Read the model definition and answer for the solid it produces. Units are mm, in the model's axes. Face numbers are marked on the shaded views. A direction names the side the tool comes from. Give positions to 0.01 mm unless a question says otherwise; leave off trailing zeros. Loops run counter-clockwise (first coordinate to the right, second up) from the corner with the lowest first, then second, coordinate; pieces in that order, holes last. Notation, with made-up numbers: (57, 65.5) -> (112, 65.5) arc R34 cw to (112, 95.5) -> close; hole circle Ø3 at (85, -7). An arc over 180 degrees is marked (long way). Write each question's results on one line, items separated by ' | '. Start each with the question number.
Item 1: Section B-B on y = 17 is taken. Write down the section's boundary in (x, z).
Item 2: Section A-A on x = -9.25 is taken. Write down the section's boundary in (y, z), and give its area (3 significant figures).
Item 3: Section C-C on x = -4 is taken. Write down the section's boundary in (y, z).
Item 4: Section D-D on y = 26 is taken. Write down the section's boundary in (x, z).
Item 5: Each of these flat-tipped pins is pushed along its axis until it touches: P1, Ø2.5, axis at x = -15.25, y = 3.25, coming from the -Z side; P2, Ø12, axis at x = 7.25, y = -18.25, coming from the +Z side; P3, Ø17.5, axis at x = -11.5, y = 23.5, coming from the +Z side. Where does it stop, or does it pass through?
Item 6: Determine the mould class of the marked faces 3, 4, 5 and 6 for opening direction Y: +Y half, -Y half, draft (parallel to the pull), parting line (faces both ways), or undercut.
Item 7: Find the intervals of material crossed by line 1 (Y direction, x = -15, z = 5.2); line 2 (X direction, y = 20, z = 5.1); line 3 (Y direction, x = 9.25, z = 1.8), in increasing order.
Item 8: Which of the six approach directions +Z, -Z, +X, -X, +Y, -Y give full straight-line access (tool end or side, diameter ignored) to the marked faces 1 and 2?
```python
from build123d import *

# Parameters (mm, degrees)
F0_W      = 38.5
F0_H      = 68.5
F1_DEPTH  = 6
F2_W      = 16
F2_H      = 16
F3_DEPTH  = 2
F5_DEPTH  = 2
F6_R      = 7.5
F7_DEPTH  = 2
F8_R      = 2
F9_DEPTH  = 8
F10_R     = 2.5
F11_DEPTH = 25
F12_R     = 2.5
F13_DEPTH = 25


with BuildPart() as f1:
    # F0 (on Top) → F1 (new body)
    with BuildSketch(Plane.XY):
        Rectangle(F0_W, F0_H)
    extrude(amount=F1_DEPTH)

    # F2 (on face) → F3 (cut)
    with BuildSketch(Plane.XY.offset(6)):
        with Locations((-9.25, 24.2511786477)):
            Rectangle(F2_W, F2_H)
        with Locations((9.25, 24.25)):
            Rectangle(F2_W, F2_H)
    extrude(amount=-F3_DEPTH, mode=Mode.SUBTRACT)

    # F4 (on face) → F5 (cut)
    with BuildSketch(Plane.XY.offset(6)):
        with BuildLine():
            Line((15.7500000197, 13.2511786477), (-15.75, 13.2511786477))
            ThreePointArc((-15.75, 13.2511786477), (-14.6893398282, 12.8118388195), (-14.25, 11.7511786477))
            ThreePointArc((-14.25, 11.7511786477), (-14.6893398282, 10.6905184759), (-15.75, 10.2511786477))
            Line((-15.75, 10.2511786477), (15.7500000167, 10.2511786477))
            ThreePointArc((15.7500000167, 10.2511786477), (14.25, 11.7511786492), (15.7500000197, 13.2511786477))
        make_face()
        with BuildLine():
            ThreePointArc((-14.25, 11.7511786477), (-14.6893398282, 12.8118388195), (-15.75, 13.2511786477))
            ThreePointArc((-15.75, 13.2511786477), (-16.8106601718, 12.8118388195), (-17.25, 11.7511786477))
            ThreePointArc((-17.25, 11.7511786477), (-16.8106601718, 10.6905184759), (-15.75, 10.2511786477))
            ThreePointArc((-15.75, 10.2511786477), (-14.6893398282, 10.6905184759), (-14.25, 11.7511786477))
        make_face()
        with BuildLine():
            ThreePointArc((17.25, 11.7511786477), (16.8106601788, 12.8118388125), (15.7500000197, 13.2511786477))
            ThreePointArc((15.7500000197, 13.2511786477), (14.25, 11.7511786492), (15.7500000167, 10.2511786477))
            ThreePointArc((15.7500000167, 10.2511786477), (16.8106601777, 10.6905184818), (17.25, 11.7511786477))
        make_face()
    extrude(amount=-F5_DEPTH, mode=Mode.SUBTRACT)

    # F6 (on face) → F7 (cut)
    with BuildSketch(Plane.XY.offset(6)):
        with Locations((7.25, -18.25)):
            Circle(F6_R)
    extrude(amount=-F7_DEPTH, mode=Mode.SUBTRACT)

    # F8 (on face) → F9 (cut)
    with BuildSketch(Plane.XY.offset(6)):
        with Locations((-15.25, 3.2511786477)):
            Circle(F8_R)
    extrude(amount=-F9_DEPTH, mode=Mode.SUBTRACT)

    # F10 (on face) → F11 (cut)
    with BuildSketch(Plane.XY.offset(4)):
        with Locations((-9.25, 24.2511786477)):
            Circle(F10_R)
    extrude(amount=-F11_DEPTH, mode=Mode.SUBTRACT)

    # F12 (on face) → F13 (cut)
    with BuildSketch(Plane.XY.offset(4)):
        with Locations((9.25, 24.25)):
            Circle(F12_R)
    extrude(amount=-F13_DEPTH, mode=Mode.SUBTRACT)


solid = f1.part
```
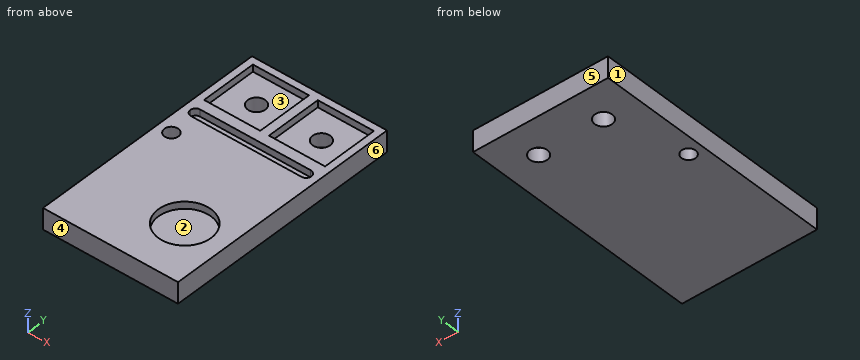
Findings:
1) outline: (-19.25, 0) -> (19.25, 0) -> (19.25, 6) -> (17.25, 6) -> (17.25, 4) -> (1.25, 4) -> (1.25, 6) -> (-1.25, 6) -> (-1.25, 4) -> (-17.25, 4) -> (-17.25, 6) -> (-19.25, 6) -> close
2) outline: (-34.25, 0) -> (21.75, 0) -> (21.75, 4) -> (16.25, 4) -> (16.25, 6) -> (13.25, 6) -> (13.25, 4) -> (10.25, 4) -> (10.25, 6) -> (-34.25, 6) -> close; (26.75, 0) -> (34.25, 0) -> (34.25, 6) -> (32.25, 6) -> (32.25, 4) -> (26.75, 4) -> close | area: 353 mm2
3) outline: (-34.25, 0) -> (34.25, 0) -> (34.25, 6) -> (32.25, 6) -> (32.25, 4) -> (16.25, 4) -> (16.25, 6) -> (13.25, 6) -> (13.25, 4) -> (10.25, 4) -> (10.25, 6) -> (-34.25, 6) -> close
4) outline: (-19.25, 0) -> (-11.04, 0) -> (-11.04, 4) -> (-17.25, 4) -> (-17.25, 6) -> (-19.25, 6) -> close; (-7.46, 0) -> (7.46, 0) -> (7.46, 4) -> (1.25, 4) -> (1.25, 6) -> (-1.25, 6) -> (-1.25, 4) -> (-7.46, 4) -> close; (11.04, 0) -> (19.25, 0) -> (19.25, 6) -> (17.25, 6) -> (17.25, 4) -> (11.04, 4) -> close
5) P1: through | P2: z = 4 | P3: z = 6
6) face 3: undercut | face 4: -Y half | face 5: +Y half | face 6: draft
7) line 1: -34.25 to 1.27, 5.24 to 10.25, 13.25 to 16.25, 32.25 to 34.25 | line 2: -19.25 to -17.25, -1.25 to 1.25, 17.25 to 19.25 | line 3: -34.25 to 21.75, 26.75 to 34.25
8) face 1: +Z, -Z, -X, +Y, -Y | face 2: +Z
